```python
from build123d import *

# Parameters (mm, degrees)
SKETCH_1_R      = 17
EXTRUDE_1_DEPTH = 75
SKETCH_2_R      = 8
EXTRUDE_2_DEPTH = 75
CHAMFER_1_SIZE  = 2
CHAMFER_2_SIZE  = 2
CHAMFER_3_SIZE  = 2


with BuildPart() as part:
    # Эскиз1 → Бобышка-Вытянуть1 (new body)
    with BuildSketch(Plane.XY):
        Circle(SKETCH_1_R)
    extrude(amount=EXTRUDE_1_DEPTH)

    # Эскиз2 → Бобышка-Вытянуть2 (add)
    with BuildSketch(Plane.XY.offset(75)):
        Circle(SKETCH_2_R)
    extrude(amount=EXTRUDE_2_DEPTH)

    # Фаска1
    chamfer_1_edges = [part.edges().sort_by_distance(p)[0] for p in [
        (-8, 0, 150),
    ]]
    chamfer(chamfer_1_edges, length=CHAMFER_1_SIZE)

    # Фаска2
    chamfer_2_edges = [part.edges().sort_by_distance(p)[0] for p in [
        (-17, 0, 75),
    ]]
    chamfer(chamfer_2_edges, length=CHAMFER_2_SIZE)

    # Фаска3
    chamfer_3_edges = [part.edges().sort_by_distance(p)[0] for p in [
        (-17, 0, 0),
    ]]
    chamfer(chamfer_3_edges, length=CHAMFER_3_SIZE)


solid = part.part
```
Check sheet for the modelled part. Datum: model origin and axes. Units: mm. A direction names the side the tool comes from. Round coordinates to 2 decimals unless told otherwise and drop trailing zeros. Order: outer loops, then holes, each group sorted by start corner. A loop starts at its lowest first (then second) coordinate and runs counter-clockwise, first axis right, second up. Notation, with made-up numbers: (19, -12) -> (66, -12) arc R15 cw to (66, 13) -> close; hole circle Ø6 at (3.25, -3.75). An arc over 180 degrees is marked (long way). Use CSV: the item, a comma, the result in double quotes.
(1) Depth check by flat-ended pin: pin 1 (4 mm diameter, centred on y = -5.5, z = 118, fed in from -X); pin 2 (6 mm diameter, centred on x = -5.5, z = 124, fed in from +Y); pin 3 (4 mm diameter, centred on x = -7, y = 13, fed in from -Z); pin 4 (12 mm diameter, centred on x = 13.5, y = 12, fed in from +Z). Enter the tip coordinate at first touch or a pass-through.
Worked out:
pin 1,"x = -7.19"
pin 2,"y = 7.6"
pin 3,"z = 0"
pin 4,"z = 75"
(2) Cross-section at D-D (z = 48). Record the boundary of the cut face in (x, y), and give its area (3 significant figures).
Worked out:
outline,"circle Ø34 at (0, 0)"
area,"908 mm²"
(3) Cross-section at A-A (y = 0). Record the boundary of the cut face in (x, z).
Worked out:
outline,"(-17, 2) -> (-15, 0) -> (15, 0) -> (17, 2) -> (17, 73) -> (15, 75) -> (8, 75) -> (8, 148) -> (6, 150) -> (-6, 150) -> (-8, 148) -> (-8, 75) -> (-15, 75) -> (-17, 73) -> close"
(4) Cross-section at C-C (z = 77). Record the boundary of the cut face in (x, y), and give its area (3 significant figures).
Worked out:
outline,"circle Ø16 at (0, 0)"
area,"201 mm²"
(5) Material ranges on line 1 along Z through (x, y) = (-4.5, 13); line 2 along Y through (x, z) = (-15, 32); line 3 along X through (y, z) = (1, 21), recorded low to high. Write a range as from..to.
Worked out:
line 1,"0..75"
line 2,"-8..8"
line 3,"-16.97..16.97"
(6) Tool access check on faces 1 (the face through (-1.73, -7.81, 110.99)), 2 (the face through (9.139, 14.334, 37.003)). Record the directions out of +Z, -Z, +X, -X, +Y, -Y that give a thin tool (end or side, any length) a straight path to the whole face; none if there is none.
Worked out:
face 1,"+Z"
face 2,"+Z, -Z"
